Geometry check sheet. Reference: the model listing, model coordinates, mm. Face numbers are marked on the shaded views. Round coordinates to 2 decimals unless told otherwise and drop trailing zeros. Loops run counter-clockwise (first coordinate to the right, second up) from the corner with the lowest first, then second, coordinate; pieces in that order, holes last. Notation, with made-up numbers: (60.25, -11) - (64.25, -11) arc R29 ccw to (64.25, 25) - close; hole circle Ø6 at (14.25, 67). An arc over 180 degrees is marked (long way). Answer as CSV lines item,"result". Start each with the question number.
1) Cross-section at D-D on y = 3.25. Record the boundary of the cut face in (x, z), and give its area (3 significant figures).
2) Cross-section at A-A on z = 20. Record the boundary of the cut face in (x, y), and give its area (3 significant figures).
3) Thickness scan on line 1 along X through (y, z) = (0, 2.9); line 2 along Y through (x, z) = (78.75, 20); line 3 along Y through (x, z) = (76.35, 29). Record the ranges inside material, lowest first.
4) Cross-section at B-B on y = -3. Record the boundary of the cut face in (x, z).
5) Depth check by flat-ended pin: P1, Ø12, axis at x = 47, y = -6, coming from the +Z side; P2, Ø2.5, axis at x = -9, y = 0, coming from the +Z side; P3, Ø15, axis at y = 4, z = 15, coming from the -X side. Enter the tip coordinate at first touch or a pass-through.
6) Draft check along Z on the marked faces 1, 2 and 3. Enter one of: released by +Z, released by -Z, zero draft, split by the parting line, or undercut.
7) Cross-section at C-C on z = 11.5. Record the boundary of the cut face in (x, y).
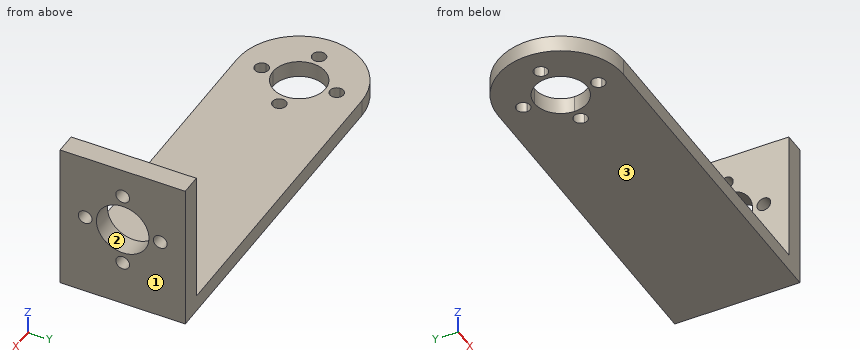
from build123d import *

# Parameters (mm, degrees)
EXTRUDE_1_DEPTH     = 4
SKETCH_2_W          = 5
SKETCH_2_H          = 30
EXTRUDE_2_DEPTH     = 36
SKETCH_4_R          = 6.3
SKETCH_4_R_2        = 1.65
CUT_EXTRUDE_1_DEPTH = 34


with BuildPart() as part:
    # 草图1 → 凸台-拉伸1 (new body)
    with BuildSketch(Plane.XY):
        with BuildLine():
            Line((0, 10.65), (0, 15))
            ThreePointArc((0, 15), (-15, 0), (0, -15))
            Line((0, -15), (0, -10.65))
            ThreePointArc((0, -10.65), (-1.219028814, -10.111966164), (-1.643053084, -8.84875))
            ThreePointArc((-1.643053084, -8.84875), (-6.363961031, -6.363961031), (-8.84875, -1.643053084))
            ThreePointArc((-8.84875, -1.643053084), (-10.65, 0), (-8.84875, 1.643053084))
            ThreePointArc((-8.84875, 1.643053084), (-6.363961031, 6.363961031), (-1.643053084, 8.84875))
            ThreePointArc((-1.643053084, 8.84875), (-1.219028814, 10.111966164), (0, 10.65))
        make_face()
        with BuildLine():
            ThreePointArc((0, 7.35), (-1.111966164, 7.780971186), (-1.643053084, 8.84875))
            ThreePointArc((-1.643053084, 8.84875), (-6.363961031, 6.363961031), (-8.84875, 1.643053084))
            ThreePointArc((-8.84875, 1.643053084), (-7.780971186, 1.111966164), (-7.35, 0))
            ThreePointArc((-7.35, 0), (-7.780971186, -1.111966164), (-8.84875, -1.643053084))
            ThreePointArc((-8.84875, -1.643053084), (-6.363961031, -6.363961031), (-1.643053084, -8.84875))
            ThreePointArc((-1.643053084, -8.84875), (-1.111966164, -7.780971186), (0, -7.35))
            Line((0, -7.35), (0, -6.3))
            ThreePointArc((0, -6.3), (-6.3, 0), (0, 6.3))
            Line((0, 6.3), (0, 7.35))
        make_face()
        with BuildLine():
            ThreePointArc((1.643053084, 8.84875), (1.111966164, 7.780971186), (0, 7.35))
            Line((0, 7.35), (0, 6.3))
            ThreePointArc((0, 6.3), (4.454772721, 4.454772721), (6.3, 0))
            ThreePointArc((6.3, 0), (4.454772721, -4.454772721), (0, -6.3))
            Line((0, -6.3), (0, -7.35))
            ThreePointArc((0, -7.35), (1.111966164, -7.780971186), (1.643053084, -8.84875))
            ThreePointArc((1.643053084, -8.84875), (6.363961031, -6.363961031), (8.84875, -1.643053084))
            ThreePointArc((8.84875, -1.643053084), (7.35, 0), (8.84875, 1.643053084))
            ThreePointArc((8.84875, 1.643053084), (6.363961031, 6.363961031), (1.643053084, 8.84875))
        make_face()
        with BuildLine():
            ThreePointArc((15, 0), (10.606601718, 10.606601718), (0, 15))
            Line((0, 15), (0, 10.65))
            ThreePointArc((0, 10.65), (1.166726189, 10.166726189), (1.65, 9))
            ThreePointArc((1.65, 9), (1.648262356, 8.924295274), (1.643053084, 8.84875))
            ThreePointArc((1.643053084, 8.84875), (6.363961031, 6.363961031), (8.84875, 1.643053084))
            ThreePointArc((8.84875, 1.643053084), (10.111966164, 1.219028814), (10.65, 0))
            ThreePointArc((10.65, 0), (10.111966164, -1.219028814), (8.84875, -1.643053084))
            ThreePointArc((8.84875, -1.643053084), (6.363961031, -6.363961031), (1.643053084, -8.84875))
            ThreePointArc((1.643053084, -8.84875), (1.648262356, -8.924295274), (1.65, -9))
            ThreePointArc((1.65, -9), (1.166726189, -10.166726189), (0, -10.65))
            Line((0, -10.65), (0, -15))
            ThreePointArc((0, -15), (10.606601718, -10.606601718), (15, 0))
        make_face()
        with BuildLine():
            Line((80, 15), (0, 15))
            ThreePointArc((0, 15), (10.606601718, 10.606601718), (15, 0))
            ThreePointArc((15, 0), (10.606601718, -10.606601718), (0, -15))
            Line((0, -15), (80, -15))
            Line((80, -15), (80, 15))
        make_face()
    extrude(amount=EXTRUDE_1_DEPTH)

    # 草图2 → 凸台-拉伸2 (add)
    with BuildSketch(Plane.XY):
        with Locations((77.5, 0)):
            Rectangle(SKETCH_2_W, SKETCH_2_H)
    extrude(amount=EXTRUDE_2_DEPTH)

    # 草图4 → 切除-拉伸1 (cut)
    with BuildSketch(Plane(origin=(80, 0, 0), x_dir=(0, 0, -1), z_dir=(1, 0, 0))):
        with Locations((-20, 0)):
            Circle(SKETCH_4_R)
        with Locations((-29, 0)):
            Circle(SKETCH_4_R_2)
        with Locations((-20, 9)):
            Circle(SKETCH_4_R_2)
        with Locations((-11, 0)):
            Circle(SKETCH_4_R_2)
        with Locations((-20, -9)):
            Circle(SKETCH_4_R_2)
    extrude(amount=-CUT_EXTRUDE_1_DEPTH, mode=Mode.SUBTRACT)


solid = part.part
Answer block:
1,outline,"(-14.64, 0) - (-5.4, 0) - (-5.4, 4) - (-14.64, 4) - close; (5.4, 0) - (80, 0) - (80, 14.6) - (75, 14.6) - (75, 4) - (5.4, 4) - close; (75, 25.4) - (80, 25.4) - (80, 36) - (75, 36) - close"
1,area,"441 mm^2"
2,outline,"(75, -15) - (80, -15) - (80, -10.65) - (75, -10.65) - close; (75, -7.35) - (80, -7.35) - (80, -6.3) - (75, -6.3) - close; (75, 6.3) - (80, 6.3) - (80, 7.35) - (75, 7.35) - close; (75, 10.65) - (80, 10.65) - (80, 15) - (75, 15) - close"
2,area,"54.0 mm^2"
3,line 1,"x = -15 to -10.65, -7.35 to -6.3, 6.3 to 7.35, 10.65 to 80"
3,line 2,"y = -15 to -10.65, -7.35 to -6.3, 6.3 to 7.35, 10.65 to 15"
3,line 3,"y = -15 to -1.65, 1.65 to 15"
4,outline,"(-14.7, 0) - (-5.54, 0) - (-5.54, 4) - (-14.7, 4) - close; (5.54, 0) - (80, 0) - (80, 14.46) - (75, 14.46) - (75, 4) - (5.54, 4) - close; (75, 25.54) - (80, 25.54) - (80, 36) - (75, 36) - close"
5,P1,"stops at z = 4"
5,P2,"passes through"
5,P3,"stops at x = 75"
6,face 1,"zero draft"
6,face 2,"undercut"
6,face 3,"released by -Z"
7,outline,"(75, -15) - (80, -15) - (80, -1.57) - (75, -1.57) - close; (75, 1.57) - (80, 1.57) - (80, 15) - (75, 15) - close"
